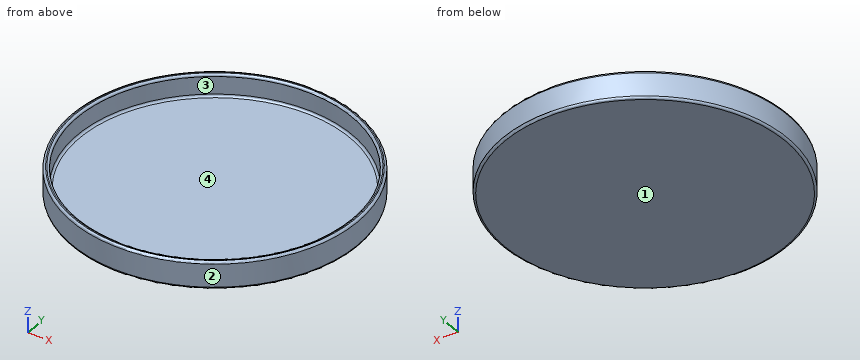
from build123d import *

# Parameters (mm, degrees)
CYLINDER001_R     = 50
CYLINDER001_DEPTH = 10
CYLINDER_R        = 52
CYLINDER_DEPTH    = 10
FILLET_R          = 0.8


with BuildPart() as cylinder001:
    # Cylinder001 → Cylinder001 (new body)
    with BuildSketch(Plane.XY.offset(2)):
        Circle(CYLINDER001_R)
    extrude(amount=CYLINDER001_DEPTH)


with BuildPart() as fillet_body:
    # Cylinder → Cylinder (new body)
    with BuildSketch(Plane.XY):
        Circle(CYLINDER_R)
    extrude(amount=CYLINDER_DEPTH)

    # Cut: cut Cylinder001
    add(cylinder001.part, mode=Mode.SUBTRACT)

    # Fillet
    fillet_edges = [fillet_body.edges().sort_by_distance(p)[0] for p in [
        (-52, 0, 10),
        (-52, 0, 0),
        (-50, 0, 10),
        (-50, 0, 2),
    ]]
    fillet(fillet_edges, radius=FILLET_R)


solid = fillet_body.part
Could you check a few things on this model? Use its own coordinates, in mm. Face numbers are marked on the shaded views. Coordinates: 2 decimals unless noted, no trailing zeros. Order: outer loops, then holes, each group sorted by start corner. A loop starts at its lowest first (then second) coordinate and runs counter-clockwise, first axis right, second up. Notation, with made-up numbers: (47, 40.5) -> (103, 40.5) arc R6 cw to (103, 45.5) -> close; hole circle Ø9 at (32, -31.75). An arc over 180 degrees is marked (long way). One line per item, written item: value. Start each with the question number.
1) I'm going to push flat-ended pins straight in: pin 1 (1 mm diameter, centred on x = -3, y = 5, fed in from +Z); pin 2 (1.5 mm diameter, centred on y = 22, z = 4.5, fed in from +X); pin 3 (6 mm diameter, centred on x = -3.5, z = 5, fed in from -Y). Where does each tip first touch, or does it pass through?
2) Imagine slicing it at B-B on z = 5.75. List the corners of the cut face in (x, y) for me.
3) Imagine slicing it at A-A on y = 0. List the corners of the cut face in (x, z) for me, plus the area to 3 significant figures.
4) We'd pull the mould along Y, two halves only. Please class the marked faces 1, 2, 3 and 4: +Y half, -Y half, draft (parallel to the pull), parting line (faces both ways), or undercut.
5) If I drill on L1, parallel to Y at x = 0, z = 7.5; L2, parallel to Z at x = 35, y = 2.5; L3, parallel to Y at x = -9, z = 8.75, over which ranges is the centre line in solid material (lowest first)? Write a range as [from, to].
Answer list:
1. pin 1: stops at z = 2
1. pin 2: stops at x = 47.46
1. pin 3: stops at y = -52
2. outline: circle Ø104 at (0, 0); hole circle Ø100 at (0, 0)
3. outline: (-52, 0.8) arc R0.8 ccw to (-51.2, 0) -> (51.2, 0) arc R0.8 ccw to (52, 0.8) -> (52, 9.2) arc R0.8 ccw to (51.2, 10) -> (50.8, 10) arc R0.8 ccw to (50, 9.2) -> (50, 2.8) arc R0.8 cw to (49.2, 2) -> (-49.2, 2) arc R0.8 cw to (-50, 2.8) -> (-50, 9.2) arc R0.8 ccw to (-50.8, 10) -> (-51.2, 10) arc R0.8 ccw to (-52, 9.2) -> close
3. area: 239 mm2
4. face 1: draft
4. face 2: parting line
4. face 3: undercut
4. face 4: undercut
5. L1: y = [-52, -50], [50, 52]
5. L2: z = [0, 2]
5. L3: y = [-51.22, -49.18], [49.18, 51.22]
